Autodesk Inventor part; units mm, degrees
ref_plane "作業平面1" through (1, 0, 0) normal (1, 0, 0) x (0, 0, -1)
ref_plane "YZ Plane" through (0, 0, 0) normal (1, 0, 0) x (0, 1, 0)
ref_plane "XZ Plane" through (0, 0, 0) normal (0, 1, 0) x (-1, 0, 0)
sketch "スケッチ1" plane through (0, 0, 0) normal (1, 0, 0) x (0, 1, 0)
  circle A0 centre (0, 0) radius 3.635
  circle A1 centre (0, 0) radius 1.635
  circle A2 centre (0, 0) radius 2.635
  dimension "d0" = 3.27
  dimension "d1" = 2
  dimension "d7" = 1
extrude "押し出し1" add sketch "スケッチ1" along normal mid plane 4 contours A0 | A2
ref_plane "作業平面1" through (1, 0, 0) normal (1, 0, 0) x (0, 0, -1)
extrude "押し出し3" cut sketch "スケッチ1" against normal blind 1 from surface at 1 contours A0
chamfer "面取り3" distance 1 angle 45 1 edges at (2, -3.635, 0)
properties part number "spacer_Φ3.2_1"
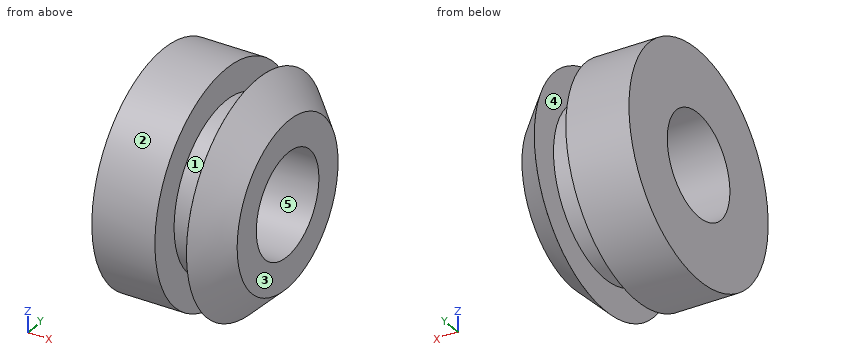
Work out the finished part from the listing and answer in its coordinate system (mm). Face numbers are marked on the shaded views. A direction names the side the tool comes from. Round coordinates to 2 decimals unless told otherwise and drop trailing zeros. Write each loop counter-clockwise with the first axis right and the second up, starting at its lowest first coordinate (ties: lowest second). Pieces come first, ordered by that corner, then holes. Notation, with made-up numbers: (-3.75, 82.5) -> (53.25, 82.5) arc R24 ccw to (53.25, 112.5) -> close; hole circle Ø2 at (72, -0.75). An arc over 180 degrees is marked (long way). Write each question's results on one line, items separated by ' | '.
Item 1: A cutting plane is placed at C-C, the plane x = -1.7. Determine the outline of the cut face in (y, z) (3 decimals), plus the area to 3 significant figures.
Result set:
outline: circle Ø7.27 at (0, 0); hole circle Ø3.27 at (0, 0) | area: 33.1 mm^2
Item 2: A flat-ended cylindrical pin translates along its axis: P1, Ø1.5, axis at x = 0.5, y = 0.5, coming from the +Z side (3 decimals). Find the tip coordinate at first contact, or state that the pin passes through.
Result set:
P1: z = 3.635
Item 3: Which of the six approach directions +Z, -Z, +X, -X, +Y, -Y give full straight-line access (tool end or side, diameter ignored) to the marked faces 1 and 2?
Result set:
face 1: none | face 2: +X, -X
Item 4: The mould has two halves that part along X. Classify the marked faces 3, 4 and 5: +X half, -X half, draft (parallel to the pull), parting line (faces both ways), or undercut.
Result set:
face 3: +X half | face 4: undercut | face 5: draft
Item 5: Find the intervals of material crossed by line 1 along Z through (x, y) = (-0.2, 0) (3 decimals); line 2 along Z through (x, y) = (0.1, 0) (3 decimals); line 3 along X through (y, z) = (3, -0.5), in increasing order. Write a range as [from, to].
Result set:
line 1: [-3.635, -1.635], [1.635, 3.635] | line 2: [-2.635, -1.635], [1.635, 2.635] | line 3: [-2, 0], [1, 1.59]
